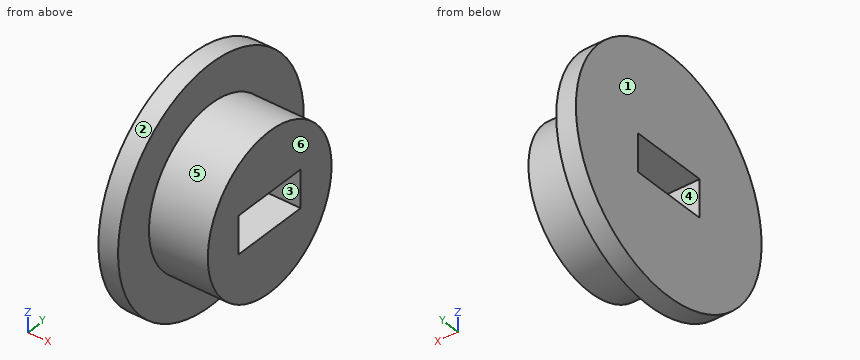
from build123d import *

# Parameters (mm, degrees)
F0_R     = 19.05
F1_DEPTH = 3.175
F2_R     = 12.7
F3_DEPTH = 9.525
F4_W     = 12.7
F4_H     = 6.096
F5_DEPTH = 12.701


with BuildPart() as f1:
    # F0 (on Right) → F1 (new body)
    with BuildSketch(Plane.YZ):
        Circle(F0_R)
    extrude(amount=F1_DEPTH)

    # F2 (on face) → F3 (join)
    with BuildSketch(Plane.YZ.offset(3.175)):
        Circle(F2_R)
    extrude(amount=F3_DEPTH)

    # F4 (on Right) → F5 (cut, through all)
    with BuildSketch(Plane.YZ):
        Rectangle(F4_W, F4_H)
    extrude(amount=F5_DEPTH, mode=Mode.SUBTRACT)


solid = f1.part
Geometry: final body of the model. Coordinates: model frame, mm. Face numbers are marked on the shaded views. A direction names the side the tool comes from. Coordinates: 2 decimals unless noted, no trailing zeros. Loops run counter-clockwise (first coordinate to the right, second up) from the corner with the lowest first, then second, coordinate; pieces in that order, holes last. Notation, with made-up numbers: M 47.25,36.25 L 60.25,36.25 A8 cw 60.25,51.25 Z; hole C -26,74 d9. An arc over 180 degrees is marked long. One line per item, written item: value. Start each with the question number.
1) Reachability of the marked faces 4, 5 and 6 from +Z, -Z, +X, -X, +Y, -Y: full face, straight path, thin tool, end or side. Return the list, or none.
2) Cut plane D-D (y = 7). Return loops of the section in (x, z) (3 decimals), then the cut area to 3 significant figures.
3) Pin query (flat end, axial travel): P1, Ø5, axis at x = 6, z = 0.5, coming from the -Y side; P2, Ø6, axis at x = 6, y = 0.5, coming from the -Z side; P3, Ø5, axis at x = 5, y = 7.5, coming from the -Z side. Return the tip coordinate at first contact, or that it passes through.
4) Cut plane C-C (x = 11.75). Return loops of the section in (y, z), then the cut area to 3 significant figures.
5) Draft query along Z for the marked faces 1, 2 and 3. Return one class per face: released by +Z, released by -Z, zero draft, split by the parting line, or undercut.
6) Material intervals for L1, parallel to Z at x = 0.5, y = 0; L2, parallel to X at y = -1, z = 17 (3 decimals); L3, parallel to Y at x = 2.5, z = 2.5, sorted ascending. Write a range as from..to.
7) Cut plane B-B (y = 0). Return loops of the section in (x, z) (3 decimals), then the cut area to 3 significant figures.
8) Cut plane A-A (z = 0). Return loops of the section in (x, y) (3 decimals).
Evaluation:
1. face 4: +X, -X
1. face 5: +X
1. face 6: +Z, -Z, +X, +Y, -Y
2. outline: M 0,-17.717 L 3.175,-17.717 L 3.175,-10.597 L 12.7,-10.597 L 12.7,10.597 L 3.175,10.597 L 3.175,17.717 L 0,17.717 Z
2. area: 314 mm^2
3. P1: y = -12.7
3. P2: z = -19.05
3. P3: z = -18.15
4. outline: C 0,0 d25.4; hole M -6.35,-3.05 L 6.35,-3.05 L 6.35,3.05 L -6.35,3.05 Z
4. area: 429 mm^2
5. face 1: zero draft
5. face 2: split by the parting line
5. face 3: undercut
6. L1: -19.05..-3.05, 3.05..19.05
6. L2: 0..3.175
6. L3: -18.89..-6.35, 6.35..18.89
7. outline: M 0,-19.05 L 3.175,-19.05 L 3.175,-12.7 L 12.7,-12.7 L 12.7,-3.048 L 0,-3.048 Z; M 0,3.048 L 12.7,3.048 L 12.7,12.7 L 3.175,12.7 L 3.175,19.05 L 0,19.05 Z
7. area: 285 mm^2
8. outline: M 0,-19.05 L 3.175,-19.05 L 3.175,-12.7 L 12.7,-12.7 L 12.7,-6.35 L 0,-6.35 Z; M 0,6.35 L 12.7,6.35 L 12.7,12.7 L 3.175,12.7 L 3.175,19.05 L 0,19.05 Z
